Geometry check sheet. Reference: the model listing, model coordinates, mm. Face numbers are marked on the shaded views. A direction names the side the tool comes from. Round coordinates to 2 decimals unless told otherwise and drop trailing zeros. Write each loop counter-clockwise with the first axis right and the second up, starting at its lowest first coordinate (ties: lowest second). Pieces come first, ordered by that corner, then holes.
Item 1: Access from +Z, -Z, +X, -X, +Y, -Y to the whole of each face (thin tool, end or side, straight path). Record for the marked faces 1, 2 and 3.
Item 2: Cross-section at B-B (z = 61). Enter the section's corners in (x, y), then the cut area to 3 significant figures.
Item 3: Cross-section at C-C (x = 76). Enter the section's corners in (y, z).
Item 4: Cross-section at A-A (y = 40). Enter the section's corners in (x, z).
Item 5: Scan lines: probe 1 along X at (y, z) = (71.5, 33); probe 2 along Y at (x, z) = (92, 39); probe 3 along Z at (x, y) = (65, 57). Record each from-to range of solid material in increasing order.
Item 6: Draft check along X on the marked faces 4, 5 and 6. Enter one of: pulls with the +X half, pulls with the -X half, needs draft (parallel to the pull), parting line crosses it, or undercut.
Item 7: Depth check by flat-ended pin: P1, Ø10, axis at x = 103.5, z = 64, coming from the -Y side; P2, Ø20, axis at y = 52.5, z = 29, coming from the +X side; P3, Ø20, axis at y = 61.5, z = 22, coming from the -X side; P4, Ø12, axis at y = 52, z = 29.5, coming from the +X side. Enter the tip coordinate at first touch or a pass-through.
Item 8: Cross-section at D-D (x = 28). Enter the section's corners in (y, z), then the cut area to 3 significant figures.
from build123d import *

# Parameters (mm, degrees)
ESQUISSE1_W             = 120
ESQUISSE1_H             = 80
BASE_EXTRUSION_DEPTH    = 3
ESQUISSE2_W             = 120
ESQUISSE2_H             = 3
BOSS_EXTRU_1_DEPTH      = 72
ENL_V_MAT_EXTRU_1_DEPTH = 3
ESQUISSE6_W             = 3
ESQUISSE6_H             = 40
BOSS_EXTRU_2_DEPTH      = 40
ENL_V_MAT_EXTRU_3_DEPTH = 3
ENL_V_MAT_EXTRU_5_DEPTH = 159.902485821
CONG_1_R                = 3


with BuildPart() as part:
    # Esquisse1 → Base-Extrusion (new body)
    with BuildSketch(Plane.XY):
        with Locations((60, 40)):
            Rectangle(ESQUISSE1_W, ESQUISSE1_H)
    extrude(amount=BASE_EXTRUSION_DEPTH)

    # Esquisse2 → Boss.-Extru.1 (add)
    with BuildSketch(Plane.XY.offset(3)):
        with Locations((60, 78.5)):
            Rectangle(ESQUISSE2_W, ESQUISSE2_H)
    extrude(amount=BOSS_EXTRU_1_DEPTH)

    # Esquisse5 → Enlèv. mat.-Extru.1 (cut)
    with BuildSketch(Plane.XY.offset(3)):
        with BuildLine():
            Line((17, 55), (17, 25))
            ThreePointArc((17, 25), (20, 22), (23, 25))
            Line((23, 25), (23, 55))
            ThreePointArc((23, 55), (20, 58), (17, 55))
        make_face()
        with BuildLine():
            Line((97, 55), (97, 25))
            ThreePointArc((97, 25), (100, 22), (103, 25))
            Line((103, 25), (103, 55))
            ThreePointArc((103, 55), (100, 58), (97, 55))
        make_face()
    extrude(amount=-ENL_V_MAT_EXTRU_1_DEPTH, mode=Mode.SUBTRACT)

    # Esquisse6 → Boss.-Extru.2 (add)
    with BuildSketch(Plane.XY.offset(3)):
        with Locations((6.5, 57)):
            Rectangle(ESQUISSE6_W, ESQUISSE6_H)
        with Locations((113.5, 57)):
            Rectangle(ESQUISSE6_W, ESQUISSE6_H)
    extrude(amount=BOSS_EXTRU_2_DEPTH)

    # Esquisse8 → Enlèv. mat.-Extru.3 (cut)
    with BuildSketch(Plane.XZ.offset(-77)):
        with BuildLine():
            Line((41.5, 64), (41.5, 58))
            ThreePointArc((41.5, 58), (44, 55.5), (46.5, 58))
            Line((46.5, 58), (46.5, 64))
            ThreePointArc((46.5, 64), (44, 66.5), (41.5, 64))
        make_face()
        with BuildLine():
            Line((73.5, 64), (73.5, 58))
            ThreePointArc((73.5, 58), (76, 55.5), (78.5, 58))
            Line((78.5, 58), (78.5, 64))
            ThreePointArc((78.5, 64), (76, 66.5), (73.5, 64))
        make_face()
    extrude(amount=-ENL_V_MAT_EXTRU_3_DEPTH, mode=Mode.SUBTRACT)

    # Esquisse10 → Enlèv. mat.-Extru.5 (cut, through all)
    with BuildSketch(Plane.ZY.offset(-5)):
        Polygon((3, 37), (43, 77), (43, 37), align=None)
    extrude(amount=-ENL_V_MAT_EXTRU_5_DEPTH, mode=Mode.SUBTRACT)

    # Congé1
    cong_1_edges = [part.edges().sort_by_distance(p)[0] for p in [
        (60, 80, 0),
    ]]
    fillet(cong_1_edges, radius=CONG_1_R)


solid = part.part
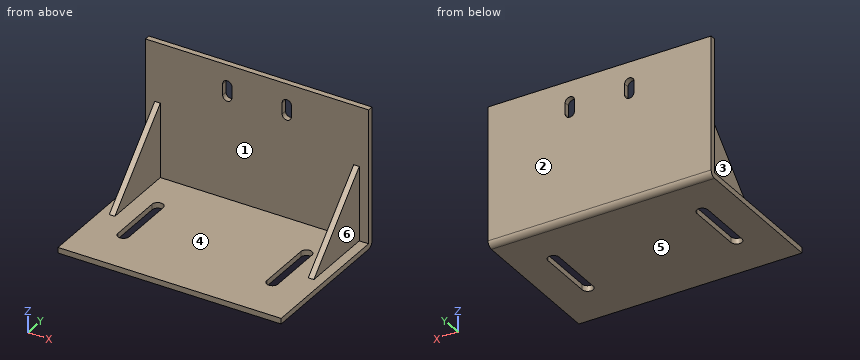
Resolved:
1. face 1: +Z, -Y
1. face 2: +Z, -Z, +X, -X, +Y
1. face 3: +Z, -X, -Y
2. outline: (0, 77) - (41.5, 77) - (41.5, 80) - (0, 80) - close; (46.5, 77) - (73.5, 77) - (73.5, 80) - (46.5, 80) - close; (78.5, 77) - (120, 77) - (120, 80) - (78.5, 80) - close
2. area: 330 mm2
3. outline: (0, 0) - (77, 0) arc R3 ccw to (80, 3) - (80, 55.5) - (77, 55.5) - (77, 3) - (0, 3) - close; (77, 66.5) - (80, 66.5) - (80, 75) - (77, 75) - close
4. outline: (0, 0) - (17, 0) - (17, 3) - (8, 3) - (8, 6) - (5, 6) - (5, 3) - (0, 3) - close; (23, 0) - (97, 0) - (97, 3) - (23, 3) - close; (103, 0) - (120, 0) - (120, 3) - (115, 3) - (115, 6) - (112, 6) - (112, 3) - (103, 3) - close
5. probe 1: x = 5 to 8, 112 to 115
5. probe 2: y = 77 to 80
5. probe 3: z = 0 to 3
6. face 4: undercut
6. face 5: needs draft
6. face 6: pulls with the +X half
7. P1: stops at y = 77
7. P2: stops at x = 115
7. P3: stops at x = 5
7. P4: passes through
8. outline: (0, 0) - (77, 0) arc R3 ccw to (80, 3) - (80, 75) - (77, 75) - (77, 3) - (0, 3) - close
8. area: 454 mm2
